Here's how the part is built. I have some questions about the finished solid (model axes, mm). A direction names the side the tool comes from. Coordinates: 2 decimals unless noted, no trailing zeros. Loops run counter-clockwise (first coordinate to the right, second up) from the corner with the lowest first, then second, coordinate; pieces in that order, holes last. Notation, with made-up numbers: (-39, 44.25) -> (-17, 44.25) arc R20 ccw to (-17, 65.25) -> close; hole circle Ø6 at (37, 80.5). An arc over 180 degrees is marked (long way). Answer as a JSON object with one key per item and string values. Group by question number.
Q1. On a 3-axis mill with a long thin cutter (end or side, diameter ignored), from which of +Z, -Z, +X, -X, +Y, -Y can I reach the whole of each face in a straight line? I mean faces 1 (the flat face through (1059.993, 282, 601)), 2 (the flat face through (1098.093, 282, 607)). Say none if no direction works.
Q2. I want a section at C-C on z = 318. Write out the boundary of the cut face in (x, y), then the cut area to 3 significant figures.
Q3. I want a section at A-A on y = 37. Write out the boundary of the cut face in (x, z), then the cut area to 3 significant figures.
Q4. I need wall thicknesses on line 1 (X direction, y = 88.9, z = 9.25) (3 decimals); line 2 (X direction, y = 88, z = 7); line 3 (Y direction, x = 152.4, z = 4.75) (3 decimals). Which ranges of each line are inside material? Lowest first, please.
Q5. I want a section at B-B on x = 131.5. Write out the boundary of the cut face in (y, z), then the cut area to 3 significant figures.
Q6. I'm going to push flat-ended pins straight in: pin 1 (4 mm diameter, centred on x = 530.5, y = 493.5, fed in from -Z); pin 2 (10 mm diameter, centred on y = 68.5, z = 379.5, fed in from -X); pin 3 (8.5 mm diameter, centred on x = 152.4, y = 88.9, fed in from +Z). Where does each tip first touch, or does it pass through?
```python
from build123d import *

# Parameters (mm, degrees)
F0_W     = 1098.0928
F0_H     = 571.5
F1_DEPTH = 12.6492
F2_W     = 38.1
F2_H     = 571.5
F3_DEPTH = 1218.2094
F5_DEPTH = 1270
F6_D     = 6.35
F6_DEPTH = 25.4
F6_TIP   = 1.9077324654


with BuildPart() as f1:
    # F0 (on Top) → F1 (new body)
    with BuildSketch(Plane.XY):
        with Locations((549.0464, 285.75)):
            Rectangle(F0_W, F0_H)
    extrude(amount=F1_DEPTH)

    # F2 (on face) → F3 (join)
    with BuildSketch(Plane.XY.offset(12.6492)):
        with Locations((1079.0428, 285.75)):
            Rectangle(F2_W, F2_H)
    extrude(amount=F3_DEPTH)

    # F4 (on face) → F5 (cut)
    with BuildSketch(Plane.XZ):
        Polygon((1059.9928, 1205.4586), (1085.3928, 1230.8586), (1059.9928, 1230.8586), align=None)
    extrude(amount=-F5_DEPTH, mode=Mode.SUBTRACT)

    # F6
    with Locations(Plane(origin=(0, 0, 0), x_dir=(1, 0, 0), z_dir=(0, 0, -1))):
        with Locations((152.4, -482.6), (907.5928, -482.6), (907.5928, -88.9), (152.4, -88.9)):
            Hole(F6_D / 2, depth=F6_DEPTH)
            with Locations((0, 0, -(F6_DEPTH + F6_TIP / 2))):  # 118° drill point
                Cone(0, F6_D / 2, F6_TIP, mode=Mode.SUBTRACT)


solid = f1.part
```
Result set:
{
 "1": {"face 1": "+Z, -X, +Y, -Y", "face 2": "+Z, -Z, +X, +Y, -Y"},
 "2": {"outline": "(1059.99, 0) -> (1098.09, 0) -> (1098.09, 571.5) -> (1059.99, 571.5) -> close", "area": "21,800 mm²"},
 "3": {"outline": "(0, 0) -> (1098.09, 0) -> (1098.09, 1230.86) -> (1085.39, 1230.86) -> (1059.99, 1205.46) -> (1059.99, 12.65) -> (0, 12.65) -> close", "area": "60,000 mm²"},
 "4": {"line 1": "x = 0 to 149.225, 155.575 to 904.418, 910.768 to 1098.093", "line 2": "x = 0 to 149.36, 155.44 to 904.55, 910.64 to 1098.09", "line 3": "y = 0 to 85.725, 92.075 to 479.425, 485.775 to 571.5"},
 "5": {"outline": "(0, 0) -> (571.5, 0) -> (571.5, 12.65) -> (0, 12.65) -> close", "area": "7,230 mm²"},
 "6": {"pin 1": "stops at z = 0", "pin 2": "stops at x = 1059.99", "pin 3": "stops at z = 12.65"}
}
